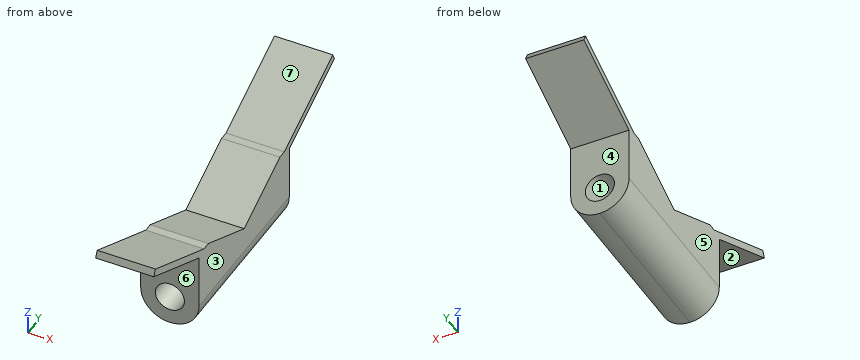
from build123d import *

# Parameters (mm, degrees)
F0_R          = 6.35
F1_DEPTH      = 38.1
F3_DEPTH      = 22.9515263319
F3_DEPTH_BACK = 2.4484736681
F5_DEPTH      = 127


with BuildPart() as f1:
    # F0 (on Front) → F1 (new body, symmetric)
    with BuildSketch(Plane.XZ):
        with BuildLine():
            Line((22.9515263319, 23.0404102315), (-2.4484736681, 23.0404102315))
            Line((-2.4484736681, 23.0404102315), (-2.4484736681, -2.3595897685))
            ThreePointArc((-2.4484736681, -2.3595897685), (1.2712702108, -11.3398458895), (10.2515263319, -15.0595897685))
            ThreePointArc((10.2515263319, -15.0595897685), (19.231782453, -11.3398458895), (22.9515263319, -2.3595897685))
            Line((22.9515263319, -2.3595897685), (22.9515263319, 23.0404102315))
        make_face()
        with Locations((10.2515263319, -2.3595897685)):
            Circle(F0_R, mode=Mode.SUBTRACT)
    extrude(amount=F1_DEPTH, both=True)

    # F2 (on Right) → F3 (join, two sides)
    with BuildSketch(Plane.YZ) as f3_sk:
        Polygon((74.8611375716, 42.0904102315), (28.7987175975, 20.6686113778), (30.1375800259, 17.7897101294), (76.2, 39.2115089832), align=None)
        Polygon((-28.7987175975, 20.6686113778), (-74.8611375716, 42.0904102315), (-76.2, 39.2115089832), (-30.1375800259, 17.7897101294), align=None)
    extrude(amount=F3_DEPTH)
    extrude(f3_sk.sketch, amount=-F3_DEPTH_BACK)

    # F4 (on Right) → F5 (cut, symmetric)
    with BuildSketch(Plane.YZ):
        Polygon((0, 9.0103000402), (37.7937594108, 26.5866738495), (-37.5799492613, 26.4872392558), align=None)
    extrude(amount=F5_DEPTH, both=True, mode=Mode.SUBTRACT)


solid = f1.part
Input: part model. Units: mm. Frame: model coordinates. Face numbers are marked on the shaded views. A direction names the side the tool comes from. Coordinates: 2 decimals unless noted, no trailing zeros. Loops run counter-clockwise (first coordinate to the right, second up) from the corner with the lowest first, then second, coordinate; pieces in that order, holes last.
(1) Section B-B on x = 12.75. Return the cut outline in (y, z).
(2) Pull-direction query (X, two-part tool) for the marked faces 1, 2 and 3; classes: released by +X, released by -X, zero draft, split by the parting line, or undercut.
(3) Section A-A on z = 34. Return the cut outline in (x, y), then the cut area to 3 significant figures.
(4) Section D-D on z = 18.5. Return the cut outline in (x, y).
(5) Set-up query: the marked faces 4, 5, 6 and 7. Return all of +Z, -Z, +X, -X, +Y, -Y with unobstructed straight access to the full face (end or side cutting, diameter ignored); none if empty.
(6) Material intervals for probe 1 along Y at (x, z) = (8.75, 16.5); probe 2 along Z at (x, y) = (10.5, -32.5); probe 3 along Y at (x, z) = (15.5, -6.5), sorted ascending.
(7) First-contact query: pin 1 Ø1 at (x, y) = (4.5, 48.5) entering from -Z; pin 2 Ø12.5 at (x, z) = (11.5, 4) entering from +Y; pin 3 Ø4 at (x, y) = (13, -33) entering from +Z. Flat tips, straight axial feed; report the tip coordinate or a pass-through.
(8) Section C-C on y = -25. Return the cut outline in (x, z).
Data:
1. outline: (-76.2, 39.21) - (-38.1, 21.49) - (-38.1, 3.48) - (38.1, 3.48) - (38.1, 21.49) - (76.2, 39.21) - (74.86, 42.09) - (33.9, 23.04) - (30.17, 23.04) - (0, 9.01) - (-30.17, 23.04) - (-33.9, 23.04) - (-74.86, 42.09) - close; (-38.1, -14.81) - (38.1, -14.81) - (38.1, -8.2) - (-38.1, -8.2) - close
2. face 1: undercut
2. face 2: zero draft
2. face 3: released by +X
3. outline: (-2.45, -64.99) - (22.95, -64.99) - (22.95, -57.46) - (-2.45, -57.46) - close; (-2.45, 57.46) - (22.95, 57.46) - (22.95, 64.99) - (-2.45, 64.99) - close
3. area: 382 mm2
4. outline: (-2.45, -38.1) - (22.95, -38.1) - (22.95, -20.41) - (-2.45, -20.41) - close; (-2.45, 20.41) - (22.95, 20.41) - (22.95, 38.1) - (-2.45, 38.1) - close
5. face 4: -Z, +X, -X, +Y
5. face 5: +Z, -Z, -X, +Y, -Y
5. face 6: -Z, +X, -X, -Y
5. face 7: +Z, +X, -X
6. probe 1: y = -38.1 to -16.1, 16.1 to 38.1
6. probe 2: z = -15.06 to -8.7, 3.99 to 23.04
6. probe 3: y = -38.1 to 38.1
7. pin 1: stops at z = 26.1
7. pin 2: stops at y = 38.1
7. pin 3: stops at z = 23.55
8. outline: (-2.45, -2.36) arc R12.7 ccw to (22.95, -2.36) - (22.95, 20.64) - (-2.45, 20.64) - close; hole circle Ø12.7 at (10.25, -2.36)
